Read the model definition and answer for the solid it produces. Units are mm, in the model's axes. Face numbers are marked on the shaded views. A direction names the side the tool comes from. Give positions to 0.01 mm unless a question says otherwise; leave off trailing zeros. Order: outer loops, then holes, each group sorted by start corner. A loop starts at its lowest first (then second) coordinate and runs counter-clockwise, first axis right, second up.
Item 1: Given pin 1 Ø10 at (x, y) = (22, 3) entering from -Z; pin 2 Ø10 at (y, z) = (7.5, 105) entering from +X; pin 3 Ø2.5 at (y, z) = (10, 16.5) entering from +X, each flat-ended and moving along its own axis, determine where each tip first touches the part or whether it passes through.
Item 2: Find the intervals of material crossed by line 1 along Y through (x, z) = (34.75, 10); line 2 along Z through (x, y) = (12, 4); line 3 along X through (y, z) = (9.5, 100.5), in increasing order.
Item 3: Which of the six approach directions +Z, -Z, +X, -X, +Y, -Y give full straight-line access (tool end or side, diameter ignored) to the marked faces 4, 5 and 6?
Item 4: A cutting plane is placed at A-A (z = 108.5). Write down the section's boundary in (x, y).
Item 5: The mould has two halves that part along Z. Classify the marked faces 1, 2 and 3: +Z half, -Z half, draft (parallel to the pull), parting line (faces both ways), or undercut.
from build123d import *

# Parameters (mm, degrees)
SKETCH_1_W          = 39.4
SKETCH_1_H          = 20
EXTRUDE_1_DEPTH     = 230
FILLET_2_RADIUS     = 10
FILLET_2_LENGTH     = 39.4
SKETCH_2_R          = 2.5
CUT_EXTRUDE_1_DEPTH = 235.205806931
SKETCH_3_W          = 10
SKETCH_3_H          = 25
CUT_EXTRUDE_2_DEPTH = 235.205806931
SKETCH_4_R          = 1.35
CUT_EXTRUDE_3_DEPTH = 20
CUT_EXTRUDE_4_DEPTH = 235.205806931
FILLET_4_R          = 2
FILLET_5_RADIUS     = 10
FILLET_5_LENGTH     = 39.4
SKETCH_6_R          = 2.1
CUT_EXTRUDE_5_DEPTH = 235.205806931
SKETCH_7_W          = 10
SKETCH_7_H          = 40
CUT_EXTRUDE_6_DEPTH = 235.205806931
CUT_EXTRUDE_7_DEPTH = 235.205806931
SKETCH_9_W          = 5
SKETCH_9_H          = 30
CUT_EXTRUDE_8_DEPTH = 235.205806931


with BuildPart() as part:
    # 草图1 → 凸台-拉伸1 (new body)
    with BuildSketch(Plane.XY):
        with Locations((19.7, 10)):
            Rectangle(SKETCH_1_W, SKETCH_1_H)
    extrude(amount=EXTRUDE_1_DEPTH)

    # 圆角2: full round fillet: the end face becomes a half cylinder, R = half its width
    fillet_2_face = Plane((19.7, 10, 0), x_dir=(1, 0, 0), z_dir=(0, 0, -1))  # on the end face: x along it, z out of the body
    fillet_2_slab = fillet_2_face.offset(-FILLET_2_RADIUS / 2) * Box(FILLET_2_LENGTH, 2 * FILLET_2_RADIUS, FILLET_2_RADIUS, mode=Mode.PRIVATE)  # the body's end, R deep
    fillet_2_round = Plane((19.7, 10, 10), x_dir=(0, 0, -1), z_dir=(1, 0, 0)) * Cylinder(FILLET_2_RADIUS, FILLET_2_LENGTH, mode=Mode.PRIVATE)  # its axis R under the face
    add(fillet_2_slab - fillet_2_round, mode=Mode.SUBTRACT)

    # 草图2 → 切除-拉伸1 (cut, through all)
    with BuildSketch(Plane.ZY):
        with Locations((10, 10)):
            Circle(SKETCH_2_R)
    extrude(amount=-CUT_EXTRUDE_1_DEPTH, mode=Mode.SUBTRACT)

    # 草图3 → 切除-拉伸2 (cut, through all)
    with BuildSketch(Plane(origin=(0, 0, 0), x_dir=(-1, 0, 0), z_dir=(0, -1, 0))):
        with Locations((-17.2, -12.5)):
            Rectangle(SKETCH_3_W, SKETCH_3_H)
    extrude(amount=-CUT_EXTRUDE_2_DEPTH, mode=Mode.SUBTRACT)

    # 草图4 → 切除-拉伸3 (cut)
    with BuildSketch(Plane(origin=(39.4, 0, 0), x_dir=(0, 0, -1), z_dir=(1, 0, 0))):
        with Locations((-3.5, 10)):
            Circle(SKETCH_4_R)
        with Locations((-10, 16.5)):
            Circle(SKETCH_4_R)
        with Locations((-16.5, 10)):
            Circle(SKETCH_4_R)
        with Locations((-10, 3.5)):
            Circle(SKETCH_4_R)
    extrude(amount=-CUT_EXTRUDE_3_DEPTH, mode=Mode.SUBTRACT)

    # 草图5 → 切除-拉伸4 (cut, through all)
    with BuildSketch(Plane(origin=(0, 0, 0), x_dir=(-1, 0, 0), z_dir=(0, -1, 0))):
        Polygon((-39.4, -45.718519933), (-29.4, -60), (-29.4, -180), (-39.4, -194.281480067), align=None)
    extrude(amount=-CUT_EXTRUDE_4_DEPTH, mode=Mode.SUBTRACT)

    # 圆角4
    fillet_4_edges = [part.edges().sort_by_distance(p)[0] for p in [
        (39.4, 10, 194.281480067),
        (34.4, 20, 52.859259966),
        (39.4, 10, 45.718519933),
        (29.4, 20, 120),
        (29.4, 10, 60),
        (34.4, 20, 187.140740034),
        (29.4, 10, 180),
        (34.4, 0, 187.140740034),
        (29.4, 0, 120),
        (34.4, 0, 52.859259966),
    ]]
    fillet(fillet_4_edges, radius=FILLET_4_R)

    # 圆角5: full round fillet: the end face becomes a half cylinder, R = half its width
    fillet_5_face = Plane((19.7, 10, 230), x_dir=(-1, 0, 0), z_dir=(0, 0, 1))  # on the end face: x along it, z out of the body
    fillet_5_slab = fillet_5_face.offset(-FILLET_5_RADIUS / 2) * Box(FILLET_5_LENGTH, 2 * FILLET_5_RADIUS, FILLET_5_RADIUS, mode=Mode.PRIVATE)  # the body's end, R deep
    fillet_5_round = Plane((19.7, 10, 220), x_dir=(0, 0, 1), z_dir=(-1, 0, 0)) * Cylinder(FILLET_5_RADIUS, FILLET_5_LENGTH, mode=Mode.PRIVATE)  # its axis R under the face
    add(fillet_5_slab - fillet_5_round, mode=Mode.SUBTRACT)

    # 草图6 → 切除-拉伸5 (cut, through all)
    with BuildSketch(Plane.ZY):
        with Locations((220, 10)):
            Circle(SKETCH_6_R)
    extrude(amount=-CUT_EXTRUDE_5_DEPTH, mode=Mode.SUBTRACT)

    # 草图7 → 切除-拉伸6 (cut, through all)
    with BuildSketch(Plane(origin=(0, 0, 0), x_dir=(-1, 0, 0), z_dir=(0, -1, 0))):
        with Locations((-15, -210)):
            Rectangle(SKETCH_7_W, SKETCH_7_H)
    extrude(amount=-CUT_EXTRUDE_6_DEPTH, mode=Mode.SUBTRACT)

    # 草图8 → 切除-拉伸7 (cut, through all)
    with BuildSketch(Plane(origin=(0, 0, 0), x_dir=(-1, 0, 0), z_dir=(0, -1, 0))):
        with BuildLine():
            Line((-5, -64), (-5, -38))
            ThreePointArc((-5, -38), (-5.878679656, -35.878679656), (-8, -35))
            Line((-8, -35), (-22.4, -35))
            ThreePointArc((-22.4, -35), (-24.521320344, -35.878679656), (-25.4, -38))
            Line((-25.4, -38), (-25.4, -52.562568091))
            ThreePointArc((-25.4, -52.562568091), (-25.261150852, -53.464685489), (-24.857456133, -54.2832974))
            Line((-24.857456133, -54.2832974), (-16.848880092, -65.720729309))
            ThreePointArc((-16.848880092, -65.720729309), (-15.776669799, -66.6610325), (-14.39142396, -67))
            Line((-14.39142396, -67), (-8, -67))
            ThreePointArc((-8, -67), (-5.878679656, -66.121320344), (-5, -64))
        make_face()
        with BuildLine():
            Line((-8, -77), (-19.4, -77))
            ThreePointArc((-19.4, -77), (-21.521320344, -77.878679656), (-22.4, -80))
            Line((-22.4, -80), (-22.4, -120.5))
            ThreePointArc((-22.4, -120.5), (-21.521320344, -122.621320344), (-19.4, -123.5))
            Line((-19.4, -123.5), (-8, -123.5))
            ThreePointArc((-8, -123.5), (-5.878679656, -122.621320344), (-5, -120.5))
            Line((-5, -120.5), (-5, -80))
            ThreePointArc((-5, -80), (-5.878679656, -77.878679656), (-8, -77))
        make_face()
        with BuildLine():
            Line((-8, -133.5), (-19.4, -133.5))
            ThreePointArc((-19.4, -133.5), (-21.521320344, -134.378679656), (-22.4, -136.5))
            Line((-22.4, -136.5), (-22.4, -177))
            ThreePointArc((-22.4, -177), (-21.521320344, -179.121320344), (-19.4, -180))
            Line((-19.4, -180), (-8, -180))
            ThreePointArc((-8, -180), (-5.878679656, -179.121320344), (-5, -177))
            Line((-5, -177), (-5, -136.5))
            ThreePointArc((-5, -136.5), (-5.878679656, -134.378679656), (-8, -133.5))
        make_face()
    extrude(amount=-CUT_EXTRUDE_7_DEPTH, mode=Mode.SUBTRACT)

    # 草图9 → 切除-拉伸8 (cut, through all)
    with BuildSketch(Plane(origin=(0, 0, 0), x_dir=(-1, 0, 0), z_dir=(0, -1, 0))):
        with Locations((-31.9, -215)):
            Rectangle(SKETCH_9_W, SKETCH_9_H)
    extrude(amount=-CUT_EXTRUDE_8_DEPTH, mode=Mode.SUBTRACT)


solid = part.part
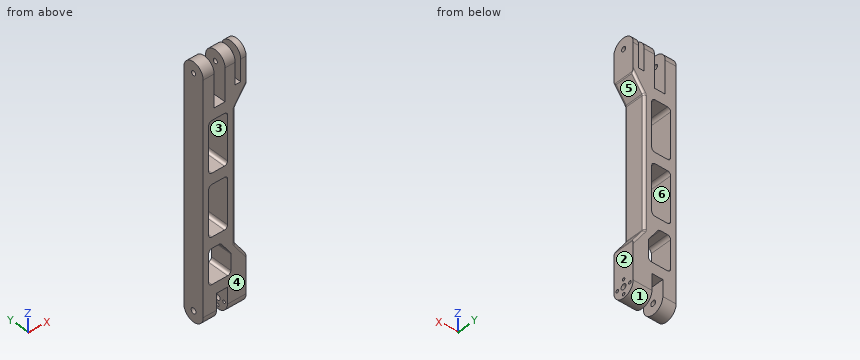
Response values:
1. pin 1: stops at z = 0.2
1. pin 2: stops at x = 29.4
1. pin 3: stops at x = 12.2
2. line 1: y = 0 to 2.15, 4.85 to 7.5, 12.5 to 15.15, 17.85 to 20
2. line 2: z = 2 to 35, 67 to 77, 123.5 to 133.5, 180 to 190
2. line 3: x = 0 to 5, 22.4 to 29.4
3. face 4: +Z, -Z, +X, -X, -Y
3. face 5: +X, +Y, -Y
3. face 6: +Y, -Y
4. outline: (0, 0) - (5, 0) - (5, 20) - (0, 20) - close; (22.4, 0) - (27.4, 0) arc R2 ccw to (29.4, 2) - (29.4, 18) arc R2 ccw to (27.4, 20) - (22.4, 20) - close
5. face 1: -Z half
5. face 2: draft
5. face 3: undercut
